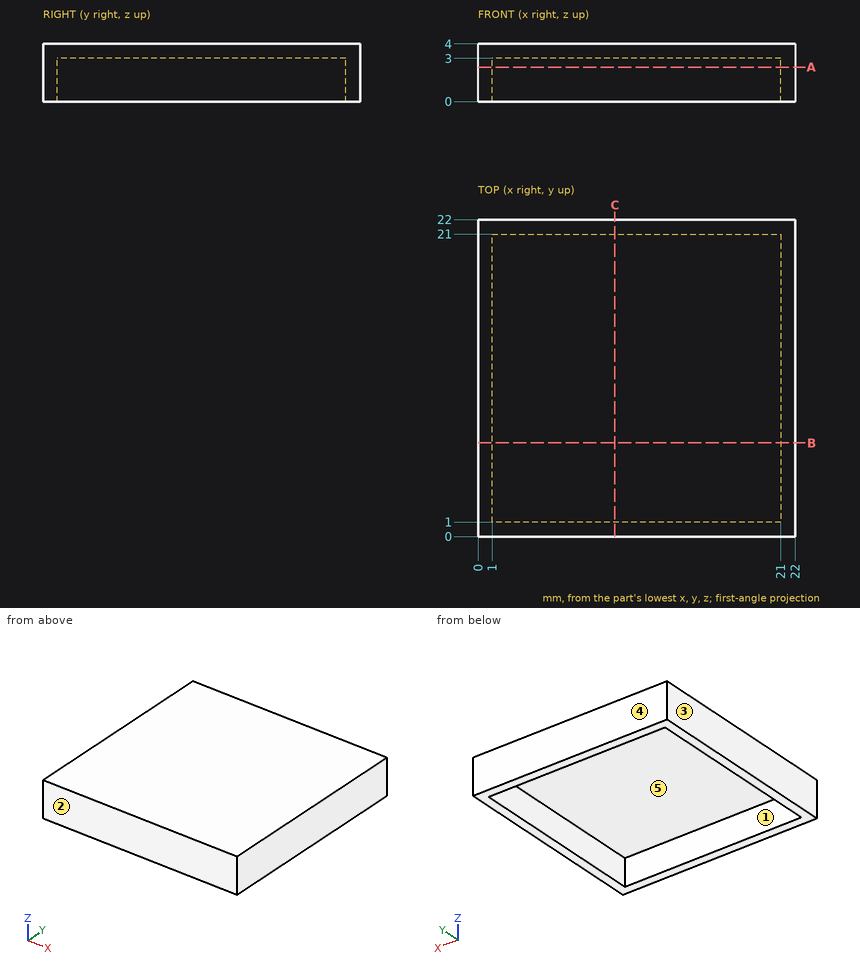
For this review, use the dimensioned drawing (mm, ordinates from the lowest corner) and the shaded views. A direction names the side the tool comes from. Give positions to 0.01 mm unless a question says otherwise; leave off trailing zeros. Order: outer loops, then holes, each group sorted by start corner. A loop starts at its lowest first (then second) coordinate and runs counter-clockwise, first axis right, second up. Notation, with made-up numbers: M 70.5,7 L 74.5,7 A29 ccw 74.5,37 Z; hole C -7,65.25 d1. An arc over 180 degrees is marked long. Use one line per item in the form item = value. Start each with the question number.
Item 1: For the marked faces 1 and 2, list the 3-axis set-ups (+Z, -Z, +X, -X, +Y, -Y) from which the entire face can be reached by the end or side of a thin tool; tool diameter is ignored.
Item 2: Insertion check: pin 1 Ø12 at (x, y) = (14, 8) entering from -Z. The pin has a flat end and moves straight along its axis. Give the tip position at first contact, or say it passes through.
Item 3: The part is to be moulded in two halves that separate along Y. For the marked faces 3, 4 and 5, say which applies: pulls with the +Y half, pulls with the -Y half, needs draft (parallel to the pull), parting line crosses it, or undercut.
Item 4: We need section A-A on z = 2.4. Give the boundary of the cut face in (x, y).
Item 5: To check wall thickness, follow line 1 along X through (y, z) = (12.75, 2.4); line 2 along Z through (x, y) = (6, 11.25). State the ranges of each line that lie inside material, in increasing order. Write a range as from..to.
Item 6: We need section B-B on y = 6.5. Give the boundary of the cut face in (x, z).
Completed:
q1.face_1 = -Z
q1.face_2 = +Z, -Z, +X, -X, -Y
q2.pin_1 = 3
q3.face_3 = needs draft
q3.face_4 = pulls with the +Y half
q3.face_5 = undercut
q4.outline = M 0,0 L 22,0 L 22,22 L 0,22 Z; hole M 1,1 L 21,1 L 21,21 L 1,21 Z
q5.line_1 = 0..1, 21..22
q5.line_2 = 3..4
q6.outline = M 0,0 L 1,0 L 1,3 L 21,3 L 21,0 L 22,0 L 22,4 L 0,4 Z
